The listing builds one solid part. Answer for the finished solid, in the listing's coordinates (mm). Coordinates: 2 decimals unless noted, no trailing zeros. Order: outer loops, then holes, each group sorted by start corner. A loop starts at its lowest first (then second) coordinate and runs counter-clockwise, first axis right, second up. Notation, with made-up numbers: (-38, -28) -> (-28, -28) arc R23 ccw to (-28, 8) -> close; hole circle Ø1 at (64, 26.25). An arc over 180 degrees is marked (long way). Return JSON: item names as keys, results as strings.
from build123d import *

# Parameters (mm, degrees)
SKETCH1_R           = 2
BOSS_EXTRUDE1_DEPTH = 4


with BuildPart() as part:
    # Sketch1 → Boss-Extrude1 (new body)
    with BuildSketch(Plane(origin=(0, 0, 0), x_dir=(1, 0, 0), z_dir=(0, 1, 0))):
        with BuildLine():
            Line((0, 3.75), (32.5, 3.75))
            ThreePointArc((32.5, 3.75), (36.25, 0), (32.5, -3.75))
            Line((32.5, -3.75), (0, -3.75))
            ThreePointArc((0, -3.75), (-3.75, 0), (0, 3.75))
        make_face()
        Circle(SKETCH1_R, mode=Mode.SUBTRACT)
        with Locations((16.25, 0)):
            Circle(SKETCH1_R, mode=Mode.SUBTRACT)
        with Locations((32.5, 0)):
            Circle(SKETCH1_R, mode=Mode.SUBTRACT)
    extrude(amount=BOSS_EXTRUDE1_DEPTH)


solid = part.part
1. The part is cut by section B-B on x = 16.25. Give the vertices of the cut face in (y, z).
Answer block:
{"outline": "(0, -3.75) -> (4, -3.75) -> (4, -2) -> (0, -2) -> close; (0, 2) -> (4, 2) -> (4, 3.75) -> (0, 3.75) -> close"}
2. Determine the mould class of faces 1 (the face through (16, 2, -3.75)), 2 (the face through (34.347, 1.972, 0.766)), 3 (the face through (16.5, 0, 2.4)) for opening direction Z: pulls with the +Z half, pulls with the -Z half, needs draft (parallel to the pull), parting line crosses it, or undercut.
Answer block:
{"face 1": "pulls with the -Z half", "face 2": "undercut", "face 3": "needs draft"}
3. The part is cut by section C-C on y = 0.6. Give the vertices of the cut face in (x, z).
Answer block:
{"outline": "(0, -3.75) -> (32.5, -3.75) arc R3.75 ccw to (32.5, 3.75) -> (0, 3.75) arc R3.75 ccw to start; hole circle Ø4 at (0, 0); hole circle Ø4 at (16.25, 0); hole circle Ø4 at (32.5, 0)"}
4. The part is cut by section A-A on z = 0. Give the vertices of the cut face in (x, y), and give its area (3 significant figures).
Answer block:
{"outline": "(-3.75, 0) -> (-2, 0) -> (-2, 4) -> (-3.75, 4) -> close; (2, 0) -> (14.25, 0) -> (14.25, 4) -> (2, 4) -> close; (18.25, 0) -> (30.5, 0) -> (30.5, 4) -> (18.25, 4) -> close; (34.5, 0) -> (36.25, 0) -> (36.25, 4) -> (34.5, 4) -> close", "area": "112 mm2"}
5. Consider line 1 (X direction, y = 1.5, z = 0); line 2 (Z direction, x = 0, y = 1.9); line 3 (Z direction, x = 15, y = 1.5). Determine where each line is inside the solid, lowest interval first. Write a range as from..to.
Answer block:
{"line 1": "x = -3.75..-2, 2..14.25, 18.25..30.5, 34.5..36.25", "line 2": "z = -3.75..-2, 2..3.75", "line 3": "z = -3.75..-1.56, 1.56..3.75"}
6. The part is cut by section D-D on z = -3. Give the vertices of the cut face in (x, y).
Answer block:
{"outline": "(-2.25, 0) -> (34.75, 0) -> (34.75, 4) -> (-2.25, 4) -> close"}
7. Each of these flat-tipped pins is pushed along its axis until it touches: pin 1 Ø3.5 at (x, z) = (32.5, 0) entering from +Y; pin 2 Ø1 at (y, z) = (1, 2) entering from -X; pin 3 Ø1 at (y, z) = (2.5, 0.5) entering from +X. Where does it stop, or does it pass through?
Answer block:
{"pin 1": "passes through", "pin 2": "stops at x = -3.44", "pin 3": "stops at x = 36.25"}
